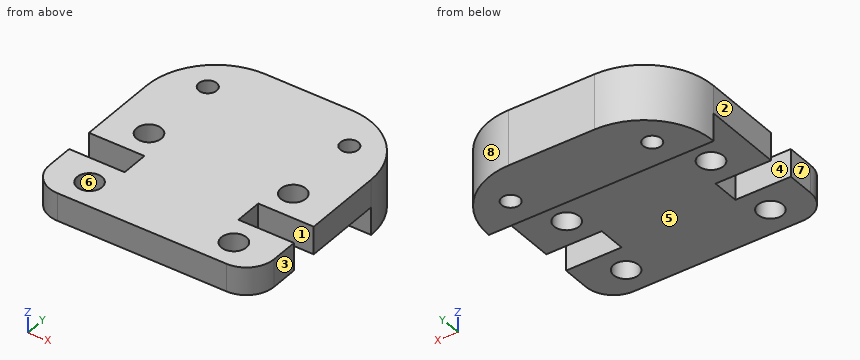
from build123d import *

# Parameters (mm, degrees)
SKETCH1_R           = 0.9
SKETCH1_R_2         = 0.65
BOSS_EXTRUDE1_DEPTH = 4
SKETCH2_W           = 16.2
SKETCH2_H           = 11.795
CUT_EXTRUDE1_DEPTH  = 2


with BuildPart() as part:
    # Sketch1 → Boss-Extrude1 (new body)
    with BuildSketch(Plane.XY):
        with BuildLine():
            Line((0, 6), (0, 11.795))
            ThreePointArc((0, 11.795), (1.464466094, 15.330533906), (5, 16.795))
            Line((5, 16.795), (11.2, 16.795))
            ThreePointArc((11.2, 16.795), (14.735533906, 15.330533906), (16.2, 11.795))
            Line((16.2, 11.795), (16.2, 6))
            Line((16.2, 6), (12.2, 6))
            Line((12.2, 6), (12.2, 4))
            Line((12.2, 4), (16.2, 4))
            Line((16.2, 4), (16.2, 2))
            ThreePointArc((16.2, 2), (15.614213562, 0.585786438), (14.2, 0))
            Line((14.2, 0), (2, 0))
            ThreePointArc((2, 0), (0.585786438, 0.585786438), (0, 2))
            Line((0, 2), (0, 4))
            Line((0, 4), (4, 4))
            Line((4, 4), (4, 6))
            Line((4, 6), (0, 6))
        make_face()
        with Locations((13.3, 2)):
            Circle(SKETCH1_R, mode=Mode.SUBTRACT)
        with Locations((13.3, 8)):
            Circle(SKETCH1_R, mode=Mode.SUBTRACT)
        with Locations((3, 13.795)):
            Circle(SKETCH1_R_2, mode=Mode.SUBTRACT)
        with Locations((13.2, 13.795)):
            Circle(SKETCH1_R_2, mode=Mode.SUBTRACT)
        with Locations((2.9, 8)):
            Circle(SKETCH1_R, mode=Mode.SUBTRACT)
        with Locations((2.9, 2)):
            Circle(SKETCH1_R, mode=Mode.SUBTRACT)
    extrude(amount=BOSS_EXTRUDE1_DEPTH)

    # Sketch2 → Cut-Extrude1 (cut)
    with BuildSketch(Plane.XY):
        with Locations((8.1, 5.8975)):
            Rectangle(SKETCH2_W, SKETCH2_H)
    extrude(amount=CUT_EXTRUDE1_DEPTH, mode=Mode.SUBTRACT)


solid = part.part
Geometry: final body of the model. Coordinates: model frame, mm. Face numbers are marked on the shaded views. A direction names the side the tool comes from. Round coordinates to 2 decimals unless told otherwise and drop trailing zeros. Loops run counter-clockwise (first coordinate to the right, second up) from the corner with the lowest first, then second, coordinate; pieces in that order, holes last. Notation, with made-up numbers: (-26.5, 18.5) -> (13.5, 18.5) arc R29 cw to (13.5, 40.5) -> close; hole circle Ø10 at (71.25, 42.5). An arc over 180 degrees is marked (long way). One line per question, with ' | ' between items. Start each with the question number.
1. Set-up query: the marked faces 1, 2, 3, 4 and 5. Return all of +Z, -Z, +X, -X, +Y, -Y with unobstructed straight access to the full face (end or side cutting, diameter ignored); none if empty.
2. Section B-B on x = 2.9. Output: boundary loops of the cut face in (y, z) (3 decimals), and give its area (3 significant figures).
3. Contact query for flat-ended pins moving along their axis: pin 1 (5 mm diameter, centred on x = 11.5, y = 8.5, fed in from -Z); pin 2 (0.6 mm diameter, centred on x = 14, z = 3, fed in from +Y); pin 3 (1 mm diameter, centred on x = 12, z = 1, fed in from -Y) (3 decimals). Output: stop coordinate, or through.
4. Section C-C on z = 3.2. Output: boundary loops of the cut face in (x, y) (3 decimals).
5. Mould query, pull axis Y, two halves, no side actions, for the marked faces 6, 7 and 8. Classes: pulls with the +Y half, pulls with the -Y half, needs draft (parallel to the pull), parting line crosses it, or undercut.
6. Section A-A on y = 8. Output: boundary loops of the cut face in (x, z), and give its area (3 significant figures).
7. Section D-D on x = 5.5. Output: boundary loops of the cut face in (y, z) (3 decimals).
8. Line query: line 1 along X through (y, z) = (2, 2.6); line 2 along Y through (x, z) = (2.75, 3.35) (3 decimals); line 3 along Z through (x, y) = (2, 3.75). Output: solid intervals per line, ascending. Write a range as [from, to].
Returned:
1) face 1: +Z, -Z, +X | face 2: +Z, -Z, -X, +Y, -Y | face 3: +Z, -Z, +X, +Y, -Y | face 4: +Z, -Z, -X | face 5: -Z, +X, -X, -Y
2) outline: (0, 2) -> (1.1, 2) -> (1.1, 4) -> (0, 4) -> close; (2.9, 2) -> (4, 2) -> (4, 4) -> (2.9, 4) -> close; (6, 2) -> (7.1, 2) -> (7.1, 4) -> (6, 4) -> close; (8.9, 2) -> (11.795, 2) -> (11.795, 0) -> (13.153, 0) -> (13.153, 4) -> (8.9, 4) -> close; (14.437, 0) -> (16.333, 0) -> (16.333, 4) -> (14.437, 4) -> close | area: 25.4 mm2
3) pin 1: stops at z = 2 | pin 2: stops at y = 16.13 | pin 3: stops at y = 11.795
4) outline: (0, 2) arc R2 ccw to (2, 0) -> (14.2, 0) arc R2 ccw to (16.2, 2) -> (16.2, 4) -> (12.2, 4) -> (12.2, 6) -> (16.2, 6) -> (16.2, 11.795) arc R5 ccw to (11.2, 16.795) -> (5, 16.795) arc R5 ccw to (0, 11.795) -> (0, 6) -> (4, 6) -> (4, 4) -> (0, 4) -> close; hole circle Ø1.8 at (2.9, 2); hole circle Ø1.8 at (2.9, 8); hole circle Ø1.3 at (3, 13.795); hole circle Ø1.8 at (13.3, 2); hole circle Ø1.8 at (13.3, 8); hole circle Ø1.3 at (13.2, 13.795)
5) face 6: undercut | face 7: needs draft | face 8: pulls with the +Y half
6) outline: (0, 2) -> (2, 2) -> (2, 4) -> (0, 4) -> close; (3.8, 2) -> (12.4, 2) -> (12.4, 4) -> (3.8, 4) -> close; (14.2, 2) -> (16.2, 2) -> (16.2, 4) -> (14.2, 4) -> close | area: 25.2 mm2
7) outline: (0, 2) -> (11.795, 2) -> (11.795, 0) -> (16.795, 0) -> (16.795, 4) -> (0, 4) -> close
8) line 1: x = [0, 2], [3.8, 12.4], [14.2, 16.2] | line 2: y = [0, 1.113], [2.887, 4], [6, 7.113], [8.887, 13.195], [14.395, 16.26] | line 3: z = [2, 4]
